```python
from build123d import *

# Parameters (mm, degrees)
F1_DEPTH    = 21
F2_START    = 2.5
F0_W        = 1
F0_H        = 1.5
F2_DEPTH    = 16
F3_SIZE     = 0.5
F4_T1_DEPTH = 20.25


# Not quite as in the source:
# - a fillet or chamfer that OpenCascade refuses, or shapes differently, is made with other operations: its cross-section is extruded or revolved along the edge and cut away or added


with BuildPart() as f1:
    # F0 (on Top) → F1 (new body)
    with BuildSketch(Plane.XY):
        Polygon((0, 2), (0, 0), (7.5, 0), (7.5, 5.25), (7.5, 6.75), (5.9, 6.75), (5.9, 2), align=None)
    extrude(amount=F1_DEPTH)

    # F0 (on Top) → F2 (join)
    with BuildSketch(Plane.XY.offset(F2_START)):
        with Locations((8, 6)):
            Rectangle(F0_W, F0_H)
    extrude(amount=F2_DEPTH)

    # F3
    f3_edges = [f1.edges().sort_by_distance(p)[0] for p in [
        (7.5, 0, 10.5),
    ]]
    chamfer(f3_edges, length=F3_SIZE)

    # F4: fillet of radius 0.85 on 2 edges, made by hand

    # F4_s2 → F4_t1 (cut)
    with BuildSketch(Plane.XY.offset(0.375)):
        with BuildLine():
            ThreePointArc((7.65, 6.75), (8.251040764, 6.501040764), (8.5, 5.9))
            Line((8.5, 5.9), (8.5, 6.75))
            Line((8.5, 6.75), (7.65, 6.75))
        make_face()
        with BuildLine():
            ThreePointArc((7.65, 5.25), (8.251040764, 5.498959236), (8.5, 6.1))
            Line((8.5, 6.1), (8.5, 5.25))
            Line((8.5, 5.25), (7.65, 5.25))
        make_face()
    extrude(amount=F4_T1_DEPTH, mode=Mode.SUBTRACT)


solid = f1.part
```
Verification items for the finished model (mm, model axes). A direction names the side the tool comes from. Round coordinates to 2 decimals unless told otherwise and drop trailing zeros. Order: outer loops, then holes, each group sorted by start corner. A loop starts at its lowest first (then second) coordinate and runs counter-clockwise, first axis right, second up.
1) Cross-section at B-B, the plane x = 2. Record the cut outline in (y, z), plus the area to 3 significant figures.
Geometry says:
outline: (0, 0) - (2, 0) - (2, 21) - (0, 21) - close
area: 42.0 mm2
2) Tool access check on faces 1 (the flat face through (8, 6, 18.5)), 2 (the flat face through (3, 2, 10)), 3 (the flat face through (8, 6, 2.5)). Record the directions out of +Z, -Z, +X, -X, +Y, -Y that give a thin tool (end or side, any length) a straight path to the whole face; none if there is none.
Geometry says:
face 1: +Z, +X, +Y, -Y
face 2: +Z, -Z, -X, +Y
face 3: -Z, +X, +Y, -Y
3) Material ranges on line 1 (Y direction, x = 5.5, z = 5); line 2 (X direction, y = 1.75, z = 7.25); line 3 (X direction, y = 4.75, z = 16.75), recorded low to high.
Geometry says:
line 1: y = 0 to 2
line 2: x = 0 to 7.5
line 3: x = 5.9 to 7.5
4) Cross-section at C-C, the plane y = 5.5. Record the cut outline in (x, z), plus the area to 3 significant figures.
Geometry says:
outline: (5.9, 0) - (7.5, 0) - (7.5, 2.5) - (8.25, 2.5) - (8.25, 18.5) - (7.5, 18.5) - (7.5, 21) - (5.9, 21) - close
area: 45.6 mm2
5) Depth check by flat-ended pin: pin 1 (2 mm diameter, centred on y = 2.5, z = 4.5, fed in from +X); pin 2 (1 mm diameter, centred on x = 4, z = 14.5, fed in from +Y); pin 3 (0.5 mm diameter, centred on x = 8, y = 5.5, fed in from -Z). Enter the tip coordinate at first touch or a pass-through.
Geometry says:
pin 1: stops at x = 7.5
pin 2: stops at y = 2
pin 3: stops at z = 2.5
6) Cross-section at A-A, the plane z = 7. Record the cut outline in (x, y), plus the area to 3 significant figures.
Geometry says:
outline: (0, 0) - (7, 0) - (7.5, 0.5) - (7.5, 5.25) - (7.65, 5.25) arc R0.85 ccw to (8.49, 6) arc R0.85 ccw to (7.65, 6.75) - (5.9, 6.75) - (5.9, 2) - (0, 2) - close
area: 23.7 mm2
7) Cross-section at D-D, the plane y = 2.5. Record the cut outline in (x, z).
Geometry says:
outline: (5.9, 0) - (7.5, 0) - (7.5, 21) - (5.9, 21) - close
